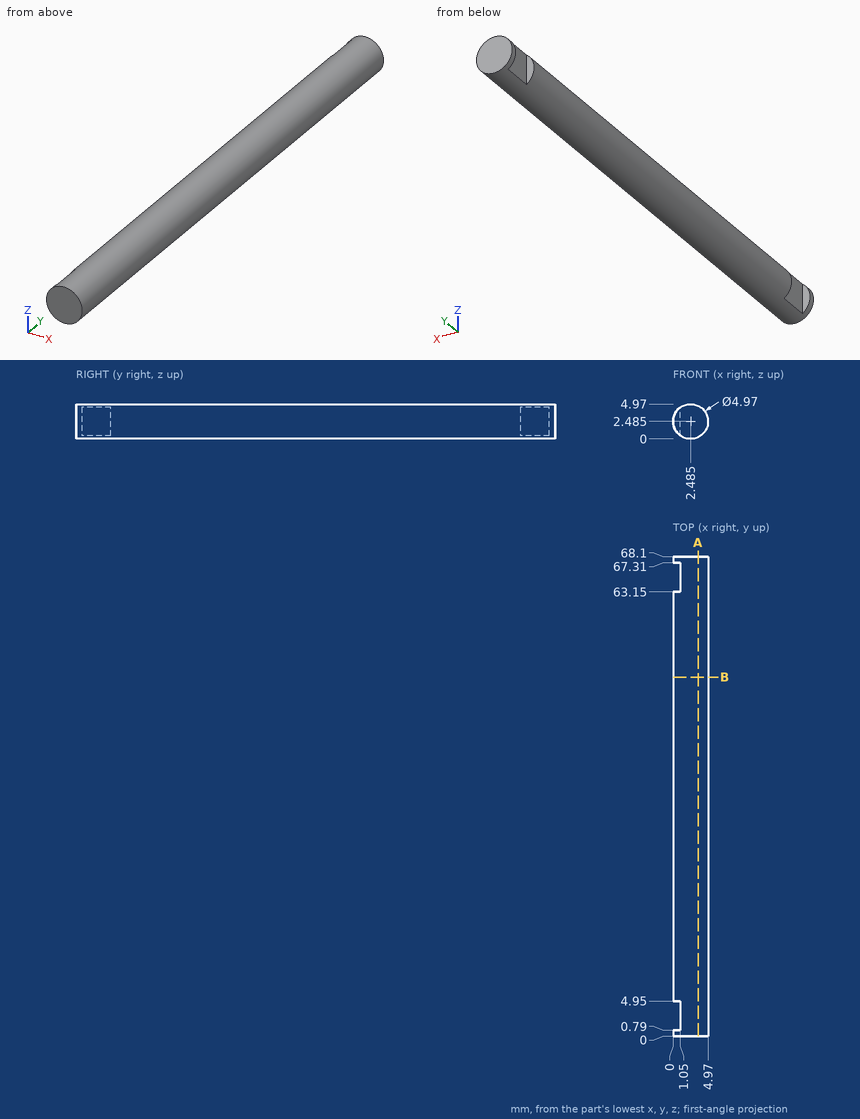
Study the drawing (mm; zero at the part's minimum x, y, z) and answer. Give positions to 0.01 mm unless a question says otherwise; leave off trailing zeros. Order: outer loops, then holes, each group sorted by start corner. A loop starts at its lowest first (then second) coordinate and runs counter-clockwise, first axis right, second up. Notation, with made-up numbers: (-37.5, 47) -> (-9.5, 47) arc R25 ccw to (-9.5, 61) -> close; hole circle Ø8 at (-25.5, 78.5). An arc over 180 degrees is marked (long way). Put each result on its own line as item: value.
Item 1: Given P1, Ø1.5, axis at x = 3.5, y = 53, coming from the +Z side; P2, Ø2, axis at x = 0.5, y = 58, coming from the +Z side; P3, Ø2, axis at y = 64.5, z = 2.5, coming from the -X side, each flat-ended and moving along its own axis, determine where each tip first touches the part or whether it passes through.
Established:
P1: stops at z = 4.96
P2: stops at z = 4.77
P3: stops at x = 1.05
Item 2: A cutting plane is placed at B-B on y = 51. Give the vertices of the cut face in (x, z) (3 decimals), plus the area to 3 significant figures.
Established:
outline: circle Ø4.97 at (2.485, 2.485)
area: 19.4 mm^2
Item 3: Straight lines are drawn through the part: line 1 (Y direction, x = 0.9, z = 2.35); line 2 (Z direction, x = 2.4, y = 36); line 3 (Z direction, x = 0.95, y = 59). For each, find the intervals that lie inside material, in ascending order.
Established:
line 1: y = 0 to 0.79, 4.95 to 63.15, 67.31 to 68.1
line 2: z = 0 to 4.97
line 3: z = 0.53 to 4.44
Item 4: A cutting plane is placed at A-A on x = 3.55. Give the vertices of the cut face in (y, z).
Established:
outline: (0, 0.24) -> (68.1, 0.24) -> (68.1, 4.73) -> (0, 4.73) -> close
